from build123d import *

# Parameters (mm, degrees)
F0_R     = 75
F2_DEPTH = 150
F1_R     = 6
F1_R_2   = 6.5
F3_DEPTH = 100
F4_W     = 120
F4_H     = 40
F5_DEPTH = 90


with BuildPart() as f2:
    # F0 (on Top) → F2 (new body)
    with BuildSketch(Plane.XY):
        with Locations((2.638103, 0)):
            Circle(F0_R)
    extrude(amount=-F2_DEPTH)

    # F1 (on face) → F3 (cut)
    with BuildSketch(Plane.XY):
        with Locations((0, 58.940991)):
            Circle(F1_R)
        with Locations((-34.644645, 47.684263)):
            Circle(F1_R)
        with Locations((-56.056213, 18.213768)):
            Circle(F1_R)
        with Locations((-56.056213, -18.213768)):
            Circle(F1_R)
        with Locations((-34.644645, -47.684263)):
            Circle(F1_R)
        with Locations((0, -58.940991)):
            Circle(F1_R)
        with Locations((34.644645, -47.684263)):
            Circle(F1_R)
        with Locations((56.056213, -18.213768)):
            Circle(F1_R)
        with Locations((56.056213, 18.213768)):
            Circle(F1_R)
        with Locations((34.644645, 47.684263)):
            Circle(F1_R)
        with Locations((0, 31.940991)):
            Circle(F1_R)
        with Locations((-24.972472, 19.914882)):
            Circle(F1_R)
        with Locations((-31.140164, -7.107539)):
            Circle(F1_R)
        with Locations((-13.858677, -28.777838)):
            Circle(F1_R)
        with Locations((13.858677, -28.777838)):
            Circle(F1_R)
        with Locations((31.140164, -7.107539)):
            Circle(F1_R)
        with Locations((24.972472, 19.914882)):
            Circle(F1_R)
        Circle(F1_R_2)
    extrude(amount=-F3_DEPTH, mode=Mode.SUBTRACT)

    # F4 (on Front) → F5 (cut)
    with BuildSketch(Plane.XZ):
        with Locations((4.467444, -120.885696)):
            Rectangle(F4_W, F4_H)
    extrude(amount=-F5_DEPTH, mode=Mode.SUBTRACT)


solid = f2.part
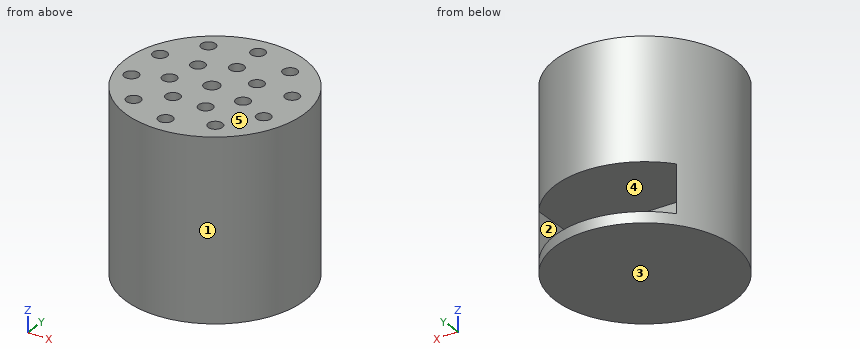
Geometry: final body of the model. Coordinates: model frame, mm. Face numbers are marked on the shaded views. A direction names the side the tool comes from. Coordinates: 2 decimals unless noted, no trailing zeros. Write each loop counter-clockwise with the first axis right and the second up, starting at its lowest first coordinate (ties: lowest second). Pieces come first, ordered by that corner, then holes. Notation, with made-up numbers: (43, 64) - (98, 64) arc R14 ccw to (98, 89) - close; hole circle Ø11 at (8.25, 40). An arc over 180 degrees is marked (long way). Return JSON: item names as keys, results as strings.
Item 1: Section query D-D (x = 57). Output: boundary loops of the cut face in (y, z), and give its area (3 significant figures).
Completed:
{"outline": "(-51.67, -150) - (51.67, -150) - (51.67, -140.89) - (0, -140.89) - (0, -100.89) - (51.67, -100.89) - (51.67, 0) - (24.14, 0) - (24.14, -100) - (12.29, -100) - (12.29, 0) - (-12.29, 0) - (-12.29, -100) - (-24.14, -100) - (-24.14, 0) - (-51.67, 0) - close", "area": "11,100 mm2"}
Item 2: Section query B-B (x = 0). Output: boundary loops of the cut face in (y, z), and give its area (3 significant figures).
Completed:
{"outline": "(-74.95, -150) - (74.95, -150) - (74.95, -140.89) - (0, -140.89) - (0, -100.89) - (74.95, -100.89) - (74.95, 0) - (64.94, 0) - (64.94, -100) - (52.94, -100) - (52.94, 0) - (37.94, 0) - (37.94, -100) - (25.94, -100) - (25.94, 0) - (6.5, 0) - (6.5, -100) - (-6.5, -100) - (-6.5, 0) - (-52.94, 0) - (-52.94, -100) - (-64.94, -100) - (-64.94, 0) - (-74.95, 0) - close", "area": "14,600 mm2"}
Item 3: Reachability of the marked faces 1 and 2 from +Z, -Z, +X, -X, +Y, -Y: full face, straight path, thin tool, end or side. Return the list, or none.
Completed:
{"face 1": "+Z, -Z", "face 2": "+Y"}
Item 4: Line query: L1, parallel to Y at x = -4.5, z = -65; L2, parallel to Y at x = 0, z = -64.5; L3, parallel to X at y = 13, z = -44.5. Output: solid intervals per line, ascending.
Completed:
{"L1": "y = -74.66 to -62.91, -54.97 to -4.69, 4.69 to 27.97, 35.91 to 54.97, 62.91 to 74.66", "L2": "y = -74.95 to -64.94, -52.94 to -6.5, 6.5 to 25.94, 37.94 to 52.94, 64.94 to 74.95", "L3": "x = -71.23 to -59.03, -53.09 to 53.09, 59.03 to 76.5"}
Item 5: Section query C-C (z = -123). Output: boundary loops of the cut face in (x, y), and give its area (3 significant figures).
Completed:
{"outline": "(-55.53, 0) - (-55.53, 47.34) arc R75 ccw (long way) to (64.47, 42.45) - (64.47, 0) - close", "area": "9,760 mm2"}
Item 6: Pull-direction query (Z, two-part tool) for the marked faces 3, 4 and 5; classes: +Z half, -Z half, draft (parallel to the pull), parting line (faces both ways), or undercut.
Completed:
{"face 3": "-Z half", "face 4": "undercut", "face 5": "+Z half"}
Item 7: Pin query (flat end, axial travel): pin 1 Ø1.5 at (x, z) = (39, -57) entering from -Y; pin 2 Ø4 at (x, z) = (-33, -33) entering from +Y; pin 3 Ø2 at (x, z) = (34.5, -62) entering from +Y. Return the tip coordinate at first contact, or that it passes through.
Completed:
{"pin 1": "stops at y = -66.01", "pin 2": "stops at y = 67.03", "pin 3": "stops at y = 68.36"}
Item 8: Section query A-A (z = -43.5). Count the separate pieces of the cut face and the enclosed holes in it, and give its area (3 significant figures).
Completed:
{"separate pieces": "1", "enclosed holes": "18", "area": "15,600 mm2"}
